Can you work these out from the drawing? Everything is in mm from the part's minimum corner. Round coordinates to 2 decimals unless told otherwise and drop trailing zeros. Loops run counter-clockwise (first coordinate to the right, second up) from the corner with the lowest first, then second, coordinate; pieces in that order, holes last. Notation, with made-up numbers: M 37,-21.75 L 64,-21.75 A15 ccw 64,-9.75 Z; hole C 26.25,54.5 d10. An arc over 180 degrees is marked long. Answer in a Markdown table with one row per item.
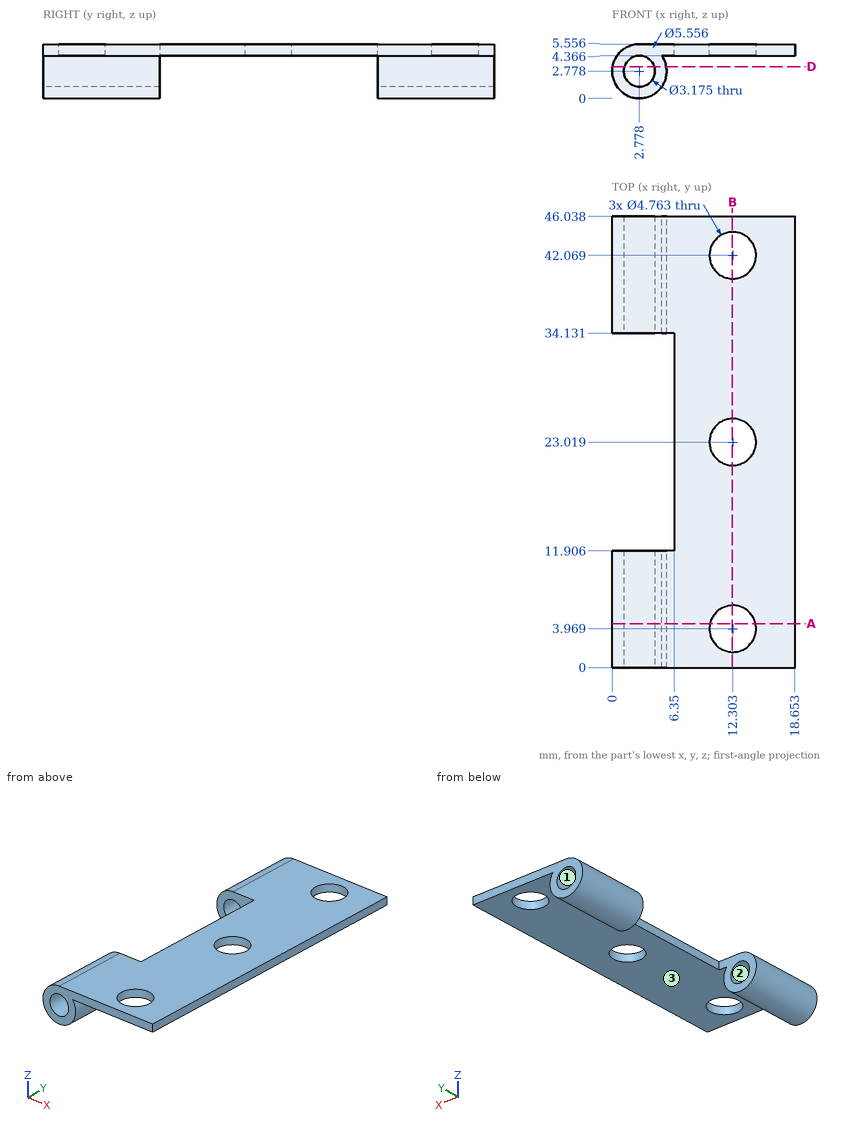
1) I want a section at D-D, the plane z = 3.25. Please give me the cut outline in (x, y) (1 decimal).
Computed:
| item | result |
|---|---|
| outline | M 0,0 L 1.3,0 L 1.3,11.9 L 0,11.9 Z; M 0,34.1 L 1.3,34.1 L 1.3,46 L 0,46 Z; M 4.3,0 L 5.5,0 L 5.5,11.9 L 4.3,11.9 Z; M 4.3,34.1 L 5.5,34.1 L 5.5,46 L 4.3,46 Z |
2) I want a section at B-B, the plane x = 12.25. State how many separate pieces and enclosed holes the cut face has.
Computed:
| item | result |
|---|---|
| separate pieces | 4 |
| enclosed holes | 0 |
3) I need wall thicknesses on line 1 (Y direction, x = 5, z = 1.55); line 2 (Z direction, x = 11, y = 18.5) (1 decimal); line 3 (X direction, y = 38, z = 0.55) (1 decimal). Which ranges of each line are inside material? Lowest first, please.
Computed:
| item | result |
|---|---|
| line 1 | y = 0 to 11.91, 34.13 to 46.04 |
| line 2 | z = 4.4 to 5.6 |
| line 3 | x = 1.1 to 4.4 |
4) I want a section at A-A, the plane y = 4.5. Please give me the cut outline in (x, z) (1 decimal).
Computed:
| item | result |
|---|---|
| outline | M 2.8,5.6 A2.8 ccw long 5.1,4.4 L 10,4.4 L 10,5.6 Z; M 14.6,4.4 L 18.7,4.4 L 18.7,5.6 L 14.6,5.6 Z; hole C 2.8,2.8 d3.2 |
5) Will these pins go through, and if not, where does the flat tip stop? P1, Ø2, axis at x = 9.5, z = 3, coming from the -Y side; P2, Ø7, axis at x = 10, y = 33.5, coming from the -Z side.
Computed:
| item | result |
|---|---|
| P1 | passes through |
| P2 | stops at z = 4.37 |
6) If we mould it in two halves opening along X, with no side actions, what happens to the marked faces 1, 2 and 3? For each: released by +X, released by -X, zero draft, split by the parting line, or undercut.
Computed:
| item | result |
|---|---|
| face 1 | undercut |
| face 2 | undercut |
| face 3 | zero draft |
